CAD build for the part. Positions are in the model's coordinates, mm. A direction names the side the tool comes from. Give positions to 0.01 mm unless a question says otherwise; leave off trailing zeros. Loops run counter-clockwise (first coordinate to the right, second up) from the corner with the lowest first, then second, coordinate; pieces in that order, holes last. Notation, with made-up numbers: M -35,61.5 L 2,61.5 A30 ccw 2,90.5 Z; hole C 38.25,25.5 d10. An arc over 180 degrees is marked long. Answer as CSV lines item,"result".
```python
from build123d import *

# Parameters (mm, degrees)
F0_W      = 88
F0_H      = 91
F1_DEPTH  = 20
F2_W      = 20
F2_H      = 91
F3_DEPTH  = 100
F5_W      = 20
F5_H      = 20
F6_DEPTH  = 70
F7_R      = 1.2
F8_DEPTH  = 25
F9_W      = 48
F9_H      = 51
F10_DEPTH = 25
F11_W     = 51
F11_H     = 80
F12_DEPTH = 88.001


with BuildPart() as f1:
    # F0 (on Top) → F1 (new body)
    with BuildSketch(Plane.XY):
        Rectangle(F0_W, F0_H)
    extrude(amount=-F1_DEPTH)

    # F2 (on face) → F3 (join)
    with BuildSketch(Plane.XY):
        with Locations((-34, 0)):
            Rectangle(F2_W, F2_H)
        with Locations((34, 0)):
            Rectangle(F2_W, F2_H)
    extrude(amount=F3_DEPTH)

    # F5 (on face) → F6 (join)
    with BuildSketch(Plane.YZ.offset(44)):
        with Locations((-35.5, 90)):
            Rectangle(F5_W, F5_H)
        with Locations((35.5, 90)):
            Rectangle(F5_W, F5_H)
    extrude(amount=-F6_DEPTH)

    # F7 (on face) → F8 (cut)
    with BuildSketch(Plane.XY.offset(100)):
        with Locations((-27, 15.5)):
            Circle(F7_R)
        with Locations((-27, -15.5)):
            Circle(F7_R)
        with Locations((27, 15.5)):
            Circle(F7_R)
        with Locations((27, -15.5)):
            Circle(F7_R)
    extrude(amount=-F8_DEPTH, mode=Mode.SUBTRACT)

    # F9 (on face) → F10 (cut)
    with BuildSketch(Plane(origin=(0, 0, -20), x_dir=(1, 0, 0), z_dir=(0, 0, -1))):
        Rectangle(F9_W, F9_H)
    extrude(amount=-F10_DEPTH, mode=Mode.SUBTRACT)

    # F11 (on face) → F12 (cut, through all)
    with BuildSketch(Plane.YZ.offset(44)):
        with Locations((0, 40)):
            Rectangle(F11_W, F11_H)
    extrude(amount=-F12_DEPTH, mode=Mode.SUBTRACT)


solid = f1.part
```
Q1. Wall check: line 1 (Y direction, x = -27, z = 88.75); line 2 (Z direction, x = -39.5, y = 12); line 3 (X direction, y = -18.5, z = 88). Give the ranges that are in metal, low to high. Write a range as [from, to].
Solution:
line 1,"y = [-45.5, -16.7], [-14.3, 14.3], [16.7, 45.5]"
line 2,"z = [-20, 0], [80, 100]"
line 3,"x = [-44, -24], [24, 44]"
Q2. Mould opens along Z. For faces 1 (the flat face through (-30, 1, 100)), 2 (the flat face through (34, 0, 80)), 3 (the flat face through (-44, -31, 39)) say: released by +Z, released by -Z, zero draft, split by the parting line, or undercut.
Solution:
face 1,"released by +Z"
face 2,"undercut"
face 3,"zero draft"
Q3. Cut at C-C (y = -32.5). Write the cut outline in (x, z).
Solution:
outline,"M -44,-20 L 44,-20 L 44,100 L -44,100 Z; hole M -24,0 L 24,0 L 24,80 L -24,80 Z"
Q4. Cut at B-B (z = 4.5). Write the cut outline in (x, y).
Solution:
outline,"M -44,-45.5 L -24,-45.5 L -24,-25.5 L -44,-25.5 Z; M -44,25.5 L -24,25.5 L -24,45.5 L -44,45.5 Z; M 24,-45.5 L 44,-45.5 L 44,-25.5 L 24,-25.5 Z; M 24,25.5 L 44,25.5 L 44,45.5 L 24,45.5 Z"
Q5. Cut at A-A (x = 17). Write the cut outline in (y, z).
Solution:
outline,"M -45.5,-20 L -25.5,-20 L -25.5,0 L -45.5,0 Z; M -45.5,80 L -25.5,80 L -25.5,100 L -45.5,100 Z; M 25.5,-20 L 45.5,-20 L 45.5,0 L 25.5,0 Z; M 25.5,80 L 45.5,80 L 45.5,100 L 25.5,100 Z"
Q6. Pin check, flat tip, straight feed: P1, Ø1.5, axis at y = 24, z = 75, coming from the -X side. Stop position of the tip, or through.
Solution:
P1,"passes through"
Q7. Cut at D-D (z = 83). Write the cut outline in (x, y).
Solution:
outline,"M -44,-45.5 L 44,-45.5 L 44,45.5 L -44,45.5 Z; hole C -27,-15.5 d2.4; hole C -27,15.5 d2.4; hole M -24,-25.5 L 24,-25.5 L 24,25.5 L -24,25.5 Z; hole C 27,-15.5 d2.4; hole C 27,15.5 d2.4"
Q8. Which spindle directions (+Z, -Z, +X, -X, +Y, -Y) get a long thin tool onto all of the face, cutting with end or side? Do faces 4 (the flat face through (24, 35, 39)), 5 (the flat face through (0, 25.5, -10)), 6 (the flat face through (-30, 45.5, 39)), 7 (the flat face through (-34, 0, 0)), 8 (the flat face through (-30, 1, -20)). Say none if no direction does.
Solution:
face 4,"+Y, -Y"
face 5,"+Z, -Z"
face 6,"+Z, -Z, +X, -X, +Y"
face 7,"+X, -X"
face 8,"-Z, +X, -X, +Y, -Y"
